Check sheet for the modelled part. Datum: model origin and axes. Units: mm. Give positions to 0.01 mm unless a question says otherwise; leave off trailing zeros. Order: outer loops, then holes, each group sorted by start corner. A loop starts at its lowest first (then second) coordinate and runs counter-clockwise, first axis right, second up.
Item 1: Release check for a two-part mould opening along X. For faces 1 (the flat face through (6.344, -0.051, 5.913)), 2 (the flat face through (-6.85, 0, 2)), 3 (the flat face through (0, 0, 0.1)) record: released by +X, released by -X, zero draft, split by the parting line, or undercut.
Item 2: Gauge pin test, flat ends, axial feed: P1, Ø2, axis at x = -5.5, z = 3, coming from the +Y side; P2, Ø1, axis at y = -2.5, z = 1.5, coming from the +X side; P3, Ø3.5, axis at x = 2.5, y = 1.5, coming from the -Z side. Record the tip position at first contact, or that the pin passes through.
Item 3: Sectioned sample at A-A on y = -0.25. Record the boundary of the cut face in (x, z), and give its area (3 significant figures).
Item 4: Sectioned sample at D-D on y = -1. Record the boundary of the cut face in (x, z).
Item 5: Sectioned sample at C-C on z = 3. Record the boundary of the cut face in (x, y), and give its area (3 significant figures).
Item 6: Sectioned sample at B-B on x = 5.25. Record the boundary of the cut face in (y, z), and give its area (3 significant figures).
Item 7: Material ranges on line 1 along Z through (x, y) = (0.25, 3.25); line 2 along X through (y, z) = (-2.25, 1.25); line 3 along Y through (x, z) = (4.5, 1.75), recorded low to high.
from build123d import *
from OCP.BRepFilletAPI import BRepFilletAPI_MakeChamfer

# Parameters (mm, degrees)
BOSS_EXTRUDE1_START = 0.1
SKETCH1_W           = 13.5
SKETCH1_H           = 7.3
BOSS_EXTRUDE1_DEPTH = 6.7
CHAMFER1_SIZE       = 1.8
CHAMFER1_SIZE2      = 0.8
BOSS_EXTRUDE2_DEPTH = 0.85
DRAFT1_ANGLE        = -3


with BuildPart() as part:
    # Sketch1 → Boss-Extrude1 (new body)
    with BuildSketch(Plane.XY.offset(BOSS_EXTRUDE1_START)):
        Rectangle(SKETCH1_W, SKETCH1_H)
    extrude(amount=BOSS_EXTRUDE1_DEPTH)

    # Chamfer1: one chamfer whose edges measure the first distance from different faces: ONE call of the kernel's chamfer builder (chamfer() names one face for all edges)
    chamfer1_edges_1 = [part.edges().sort_by_distance(p)[0] for p in [
        (6.75, 0, 6.8),
    ]]
    chamfer1_side_1 = [part.faces().sort_by_distance(p)[0] for p in [
        (6.75, 0, 3.45),
    ]]
    chamfer1_edges_2 = [part.edges().sort_by_distance(p)[0] for p in [
        (-6.75, 0, 6.8),
    ]]
    chamfer1_side_2 = [part.faces().sort_by_distance(p)[0] for p in [
        (-6.75, 0, 3.45),
    ]]
    chamfer1 = BRepFilletAPI_MakeChamfer(part.part.solid().wrapped)
    for e in chamfer1_edges_1:
        chamfer1.Add(CHAMFER1_SIZE, CHAMFER1_SIZE2, e.wrapped, chamfer1_side_1[0].wrapped)  # the first distance lies on this face
    for e in chamfer1_edges_2:
        chamfer1.Add(CHAMFER1_SIZE, CHAMFER1_SIZE2, e.wrapped, chamfer1_side_2[0].wrapped)  # the first distance lies on this face
    add(Compound.cast(chamfer1.Shape()), mode=Mode.REPLACE)

    # Sketch2 → Boss-Extrude2 (add, symmetric)
    with BuildSketch(Plane(origin=(0, 0, 0), x_dir=(1, 0, 0), z_dir=(0, 1, 0))):
        Polygon((4.35, -0.1), (6.75, -0.1), (6.75, -4.5), (6.85, -4.5), (6.85, 0), (4.35, 0), align=None)
    boss_extrude2 = extrude(amount=BOSS_EXTRUDE2_DEPTH, both=True)

    # Mirror1: Boss-Extrude2 across plane
    add(boss_extrude2.mirror(Plane(origin=(0, 0, 0), x_dir=(0, 0, 1), z_dir=(1, 0, 0))))

    # Draft1
    draft1_faces = [part.faces().sort_by_distance(p)[0] for p in [
        (0, 3.65, 3.405510617),
        (0, -3.65, 3.405510617),
    ]]
    draft(draft1_faces, Plane.XY.offset(6.8), DRAFT1_ANGLE)


solid = part.part
Report:
1. face 1: released by +X
1. face 2: released by -X
1. face 3: undercut
2. P1: stops at y = 3.5
2. P2: stops at x = 6.75
2. P3: stops at z = 0.1
3. outline: (-6.85, 0) - (-4.35, 0) - (-4.35, 0.1) - (4.35, 0.1) - (4.35, 0) - (6.85, 0) - (6.85, 4.5) - (6.75, 4.5) - (6.75, 5) - (5.95, 6.8) - (-5.95, 6.8) - (-6.75, 5) - (-6.75, 4.5) - (-6.85, 4.5) - close
3. area: 90.4 mm2
4. outline: (-6.75, 0.1) - (6.75, 0.1) - (6.75, 5) - (5.95, 6.8) - (-5.95, 6.8) - (-6.75, 5) - close
5. outline: (-6.85, -0.85) - (-6.75, -0.85) - (-6.75, -3.45) - (6.75, -3.45) - (6.75, -0.85) - (6.85, -0.85) - (6.85, 0.85) - (6.75, 0.85) - (6.75, 3.45) - (-6.75, 3.45) - (-6.75, 0.85) - (-6.85, 0.85) - close
5. area: 93.5 mm2
6. outline: (-3.65, 6.8) - (-3.3, 0.1) - (-0.85, 0.1) - (-0.85, 0) - (0.85, 0) - (0.85, 0.1) - (3.3, 0.1) - (3.65, 6.8) - close
6. area: 46.7 mm2
7. line 1: z = 0.1 to 6.8
7. line 2: x = -6.75 to 6.75
7. line 3: y = -3.39 to 3.39
